Autodesk Inventor part; units mm, degrees
ref_plane "Work Plane1" through (0, 500, 0) normal (0, -1, 0) x (1, 0, 0)
ref_plane "YZ Plane" through (0, 0, 0) normal (1, 0, 0) x (0, 1, 0)
ref_plane "XZ Plane" through (0, 0, 0) normal (0, 1, 0) x (-1, 0, 0)
sketch "Sketch1" plane through (0, 0, 0) normal (0, 1, 0) x (-1, 0, 0)
  line L0 (-12, 14) -> (12, 14) construction
  line L1 (14, 12) -> (14, -12) construction
  line L2 (12, -14) -> (-12, -14) construction
  line L3 (-14, -12) -> (-14, 12) construction
  line L4 (-14, 14) -> (14, -14) construction
  line L5 (14, 14) -> (-14, -14) construction
  arc A0 (14, 12) -> (12, 14) centre (12, 12) ccw construction
  arc A1 (12, -14) -> (14, -12) centre (12, -12) ccw construction
  arc A2 (-14, -12) -> (-12, -14) centre (-12, -12) ccw construction
  arc A3 (-12, 14) -> (-14, 12) centre (-12, 12) ccw construction
  line L6 (-12, -15) -> (12, -15)
  arc A4 (12, -15) -> (15, -12) centre (12, -12) ccw
  line L7 (15, -12) -> (15, 12)
  arc A5 (15, 12) -> (12, 15) centre (12, 12) ccw
  line L8 (12, 15) -> (-12, 15)
  arc A6 (-12, 15) -> (-15, 12) centre (-12, 12) ccw
  line L9 (-15, 12) -> (-15, -12)
  arc A7 (-15, -12) -> (-12, -15) centre (-12, -12) ccw
  line L10 (13, -12) -> (13, 12)
  arc A8 (13, 12) -> (12, 13) centre (12, 12) ccw
  line L11 (12, 13) -> (-12, 13)
  arc A9 (-12, 13) -> (-13, 12) centre (-12, 12) ccw
  line L12 (-13, 12) -> (-13, -12)
  arc A10 (-13, -12) -> (-12, -13) centre (-12, -12) ccw
  line L13 (-12, -13) -> (12, -13)
  arc A11 (12, -13) -> (13, -12) centre (12, -12) ccw
  point P0 (0, 0)
  point P1 (0, 0)
  point P2 (0, 0)
  dimension "d10" = 2
  dimension "depth" = 30
  dimension "width" = 30
  dimension "thickness" = 2
extrude "Extrusion1" add sketch "Sketch1" along normal blind 1000
ref_plane "Work Plane1" through (0, 500, 0) normal (0, -1, 0) x (1, 0, 0)
sketch "Sketch5" plane through (12, 0, -15) normal (0, 0, -1) x (-1, 0, 0)
  arc A0 (-603, 460) -> (-603, 2430) centre (-603, 1445) ccw
  line L0 (27, 0) -> (27, 1000)
  line L1 (-3, 0) -> (-3, 1000)
  line L2 (0, 0) -> (24, 0)
  line L3 (0, 0) -> (-3, 0)
  line L4 (27, 0) -> (24, 0)
  point P0 (12, 0)
  point P1 (27, 687.8177)
  point P2 (-3, 663.831)
extrude "Extrusion4" cut sketch "Sketch5" against normal through all
equation "\"d10\" = thickness"
properties part number "podest duzy profil 5" material "Steel"
Work out the finished part from the listing and answer in its coordinate system (mm). A direction names the side the tool comes from. Coordinates: 2 decimals unless noted, no trailing zeros. Write each loop counter-clockwise with the first axis right and the second up, starting at its lowest first coordinate (ties: lowest second). Pieces come first, ordered by that corner, then holes.
1. The part is cut by section A-A, the plane z = 5. Write down the section's boundary in (x, y).
Results list:
outline: (-15, 687.82) arc R985 ccw to (-13, 686.16) - (-13, 1000) - (-15, 1000) - close; (13, 665.37) arc R985 ccw to (15, 663.83) - (15, 1000) - (13, 1000) - close
2. For faces 4 (the flat face through (0, 831, 13)), 5 (the flat face through (-15, 842, 0)), determine the directions among +Z, -Z, +X, -X, +Y, -Y from which every point of the face is accessible in a straight line to the end or side of a thin tool.
Results list:
face 4: +Y, -Y
face 5: +Z, -Z, -X, +Y, -Y
3. Consider line 1 along Z through (x, y) = (-2, 924.5); line 2 along Z through (x, y) = (-12.5, 942.5). Determine where each line is inside the solid, lowest interval first.
Results list:
line 1: z = -15 to -13, 13 to 15
line 2: z = -14.96 to -12.87, 12.87 to 14.96
4. The part is cut by section B-B, the plane x = 3.5. Write down the section's boundary in (y, z), and give its area (3 significant figures).
Results list:
outline: (672.8, -15) - (1000, -15) - (1000, -13) - (672.8, -13) - close; (672.8, 13) - (1000, 13) - (1000, 15) - (672.8, 15) - close
area: 1,310 mm2
5. For a pull along X with two mould halves and no side action, classify faces 1 (the flat face through (0, 831, 15)), 2 (the flat face through (13, 830, 0)), 3 (the flat face through (15, 830, 0)) as +X half, -X half, draft (parallel to the pull), parting line (faces both ways), or undercut.
Results list:
face 1: draft
face 2: undercut
face 3: +X half
6. The part is cut by section C-C, the plane y = 780.5. Write down the section's boundary in (x, z).
Results list:
outline: (-15, -12) arc R3 ccw to (-12, -15) - (12, -15) arc R3 ccw to (15, -12) - (15, 12) arc R3 ccw to (12, 15) - (-12, 15) arc R3 ccw to (-15, 12) - close; hole (-13, -12) arc R1 ccw to (-12, -13) - (12, -13) arc R1 ccw to (13, -12) - (13, 12) arc R1 ccw to (12, 13) - (-12, 13) arc R1 ccw to (-13, 12) - close
